```python
from build123d import *

# Parameters (mm, degrees)
F0_W     = 2715.0481939316
F0_H     = 1663.144826889
F0_W_2   = 810.2502822876
F0_H_2   = 1606.2853336334
F0_H_3   = 1691.5745735168
F0_W_3   = 1165.6231880188
F0_W_4   = 2786.1232757568
F0_H_4   = 1663.1445884705
F1_DEPTH = 101.6
F2_DEPTH = 25.4
F4_DEPTH = 152.4
F5_SCALE = 0.01


with BuildPart() as f1:
    # F0 (on Front) → F1 (new body)
    with BuildSketch(Plane.XZ):
        Polygon((0, 8026.4), (0, 0), (6934.2, 0), (6934.2, 2333.8942527771), (7960.1616859436, 2333.8942527771), (7960.1616859436, 0), (8614.0480041504, 0), (8614.0480041504, 3286.2932682037), (12963.8109207153, 3286.2932682037), (12963.8109207153, 0), (13868.4, 0), (13868.4, 8026.4), (13360.4, 8026.4), (13360.4, 8382), (11379.2, 8636), (9398, 8382), (9398, 8026.4), (4470.4, 8026.4), (4470.4, 8382), (2489.2, 8636), (508, 8382), (508, 8026.4), align=None)
        with Locations((2793.0410504341, 2540.0103330612)):
            Rectangle(F0_W, F0_H, mode=Mode.SUBTRACT)
        with Locations((5962.9664421082, 2511.5805864334)):
            Rectangle(F0_W_2, F0_H_2, mode=Mode.SUBTRACT)
        with Locations((2793.0410504341, 5354.562997818)):
            Rectangle(F0_W, F0_H_3, mode=Mode.SUBTRACT)
        with Locations((5785.2799892426, 5354.562997818)):
            Rectangle(F0_W_3, F0_H_3, mode=Mode.SUBTRACT)
        with Locations((11130.0868988037, 5198.1990337372)):
            Rectangle(F0_W_4, F0_H_4, mode=Mode.SUBTRACT)
        with Locations((11130.0868988037, 5198.1990337372)):
            Rectangle(F0_W_4, F0_H_4)
    extrude(amount=-F1_DEPTH)

    # F0 (on Front) → F2 (cut)
    with BuildSketch(Plane.XZ):
        with Locations((11130.0868988037, 5198.1990337372)):
            Rectangle(F0_W_4, F0_H_4)
    extrude(amount=-F2_DEPTH, mode=Mode.SUBTRACT)

    # F3 (on Right) → F4 (join)
    with BuildSketch(Plane.YZ):
        Polygon((0, 8026.4), (0, 0), (17780, 0), (17780, 8026.4), (8907.9284667969, 8026.4), (8907.9284667969, 9539.3447875977), (5817.1215057373, 9539.3447875977), (5817.1215057373, 8026.4), align=None)
    extrude(amount=F4_DEPTH)


with BuildPart() as f1_1:
    # F5: moved
    add(f1.part.scale(F5_SCALE))


solid = f1_1.part
```
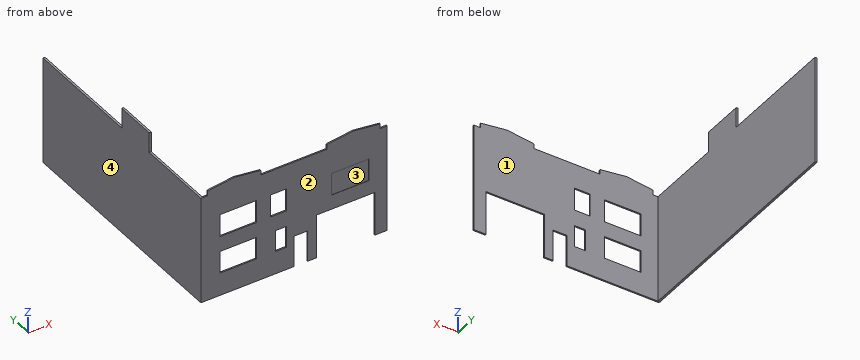
Here's how the part is built. I have some questions about the finished solid (model axes, mm). Face numbers are marked on the shaded views. A direction names the side the tool comes from. Give positions to 0.01 mm unless a question says otherwise; leave off trailing zeros. Order: outer loops, then holes, each group sorted by start corner. A loop starts at its lowest first (then second) coordinate and runs counter-clockwise, first axis right, second up. Notation, with made-up numbers: (-35, 25) - (6, 25) arc R18 cw to (6, 33) - close; hole circle Ø11 at (18.25, 3.5). An arc over 180 degrees is marked (long way). Answer as a JSON object with one key per item and string values. Group by question number.
Item 1: If we section it at A-A on z = 10: Please give me the cut outline in (x, y), and give its area (3 significant figures).
Item 2: If we section it at B-B on z = 30: Please give me the cut outline in (x, y).
Item 3: Which directions (+Z, -Z, +X, -X, +Y, -Y) give clear straight access to the entire face, cutting with the end or side of a thin tool? Please do the marked faces 1 and 2.
Item 4: If we section it at D-D on x = 120.5: Please give me the cut outline in (y, z), and give its area (3 significant figures).
Item 5: Please list where these lines run through material, in increasing order: probe 1 along X at (y, z) = (138, 64); probe 2 along Y at (x, z) = (16.5, 65).
Item 6: For P1, Ø12, axis at x = 74.5, z = 15.5, coming from the +Y side; P2, Ø1.1, axis at x = 61.5, y = 1, coming from the +Z side; P3, Ø1.1, axis at x = 33.5, y = 0.5, coming from the +Z side, each with a flat end and sliding along its axis, tell me the tip position at first contact or that it passes through.
Item 7: If we section it at C-C on x = 20: Please give me the cut outline in (y, z).
Item 8: If we mould it in two halves opening along Z, with no side actions, what happens to the marked faces 3 and 4? For each: pulls with the +Z half, pulls with the -Z half, needs draft (parallel to the pull), parting line crosses it, or undercut.
Result set:
{
 "1": {"outline": "(0, 0) - (69.34, 0) - (69.34, 1.02) - (1.52, 1.02) - (1.52, 177.8) - (0, 177.8) - close; (79.6, 0) - (86.14, 0) - (86.14, 1.02) - (79.6, 1.02) - close; (129.64, 0) - (138.68, 0) - (138.68, 1.02) - (129.64, 1.02) - close", "area": "356 mm²"},
 "2": {"outline": "(0, 0) - (14.36, 0) - (14.36, 1.02) - (1.52, 1.02) - (1.52, 177.8) - (0, 177.8) - close; (41.51, 0) - (55.58, 0) - (55.58, 1.02) - (41.51, 1.02) - close; (63.68, 0) - (86.14, 0) - (86.14, 1.02) - (63.68, 1.02) - close; (129.64, 0) - (138.68, 0) - (138.68, 1.02) - (129.64, 1.02) - close"},
 "3": {"face 1": "+Z, -Z, +X, +Y", "face 2": "+Z, -Z, +X, -X, -Y"},
 "4": {"outline": "(0, 32.86) - (1.02, 32.86) - (1.02, 85.5) - (0, 85.5) - (0, 60.3) - (0.25, 60.3) - (0.25, 43.67) - (0, 43.67) - close", "area": "49.3 mm²"},
 "5": {"probe 1": "0 to 1.52", "probe 2": "0 to 1.02"},
 "6": {"P1": "y = 1.02", "P2": "z = 80.26", "P3": "z = 85.33"},
 "7": {"outline": "(0, 0) - (1.02, 0) - (1.02, 17.08) - (0, 17.08) - close; (0, 33.72) - (1.02, 33.72) - (1.02, 45.09) - (0, 45.09) - close; (0, 62) - (1.02, 62) - (1.02, 85.73) - (0, 85.73) - close"},
 "8": {"face 3": "undercut", "face 4": "needs draft"}
}
